Part model, mm, in its own coordinate system. Give positions to 0.01 mm unless a question says otherwise; leave off trailing zeros. Order: outer loops, then holes, each group sorted by start corner. A loop starts at its lowest first (then second) coordinate and runs counter-clockwise, first axis right, second up. Notation, with made-up numbers: M -31.75,37 L 24.25,37 A24 ccw 24.25,50 Z; hole C 75.25,31 d10. An arc over 180 degrees is marked long. Return JSON: item names as keys, results as strings.
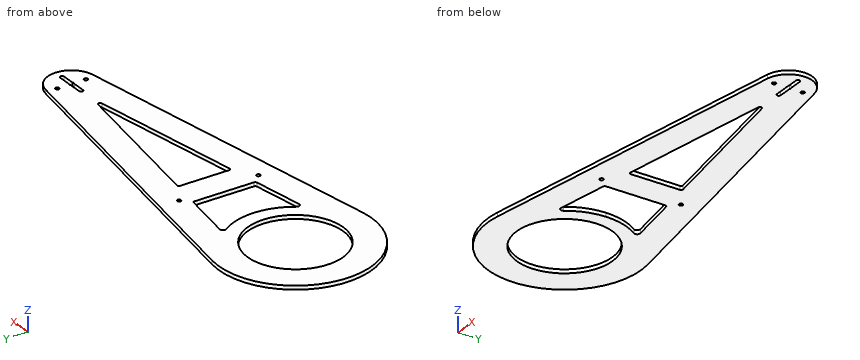
from build123d import *

# Parameters (mm, degrees)
SM_BASE_FLANGE_1_DEPTH = 4
SKETCH_6_R             = 20
SKETCH_6_R_2           = 2.5
CUT_EXTRUDE_1_DEPTH    = 10
SKETCH_7_R             = 2
CUT_EXTRUDE_2_DEPTH    = 10
CUT_EXTRUDE_3_DEPTH    = 10
SKETCH_9_R             = 2
CUT_EXTRUDE_4_DEPTH    = 80
FILLET_2_R             = 2
SKETCH_10_R            = 50
CUT_EXTRUDE_5_DEPTH    = 10


# Sheet-metal steps are written as plain solids
with BuildPart() as part:
    # Sketch 1 → 基体-法兰1 (new body)
    with BuildSketch(Plane.XY):
        with BuildLine():
            Line((12.571428571, 79.00607055), (353.928571429, 24.689397047))
            ThreePointArc((353.928571429, 24.689397047), (375, 0), (353.928571429, -24.689397047))
            Line((353.928571429, -24.689397047), (12.571428571, -79.00607055))
            ThreePointArc((12.571428571, -79.00607055), (-80, 0), (12.571428571, 79.00607055))
        make_face()
    extrude(amount=-SM_BASE_FLANGE_1_DEPTH)

    # 草图6 → 切除-拉伸1 (cut)
    with BuildSketch(Plane.XY):
        Circle(SKETCH_6_R)
        with Locations((350, 0)):
            Circle(SKETCH_6_R_2)
    extrude(amount=-CUT_EXTRUDE_1_DEPTH, mode=Mode.SUBTRACT)

    # 草图7 → 切除-拉伸2 (cut)
    with BuildSketch(Plane.XY):
        with Locations((365, 0)):
            Circle(SKETCH_7_R)
        with Locations((350, -15)):
            Circle(SKETCH_7_R)
        with Locations((335, 0)):
            Circle(SKETCH_7_R)
        with Locations((350, 15)):
            Circle(SKETCH_7_R)
        with BuildLine():
            Line((111.294862901, 32.919806827), (111.294862901, -32.919806827))
            Line((111.294862901, -32.919806827), (56.389238276, -41.656377743))
            ThreePointArc((56.389238276, -41.656377743), (53.378656764, -40.291367953), (53.450847511, -36.986577299))
            ThreePointArc((53.450847511, -36.986577299), (62.032293151, -19.416348946), (64.999939097, -0.088979461))
            ThreePointArc((64.999939097, -0.088979461), (62.058814357, 19.33141383), (53.450847511, 36.986577299))
            ThreePointArc((53.450847511, 36.986577299), (53.378656764, 40.291367953), (56.389238276, 41.656377743))
            Line((56.389238276, 41.656377743), (111.294862901, 32.919806827))
        make_face()
        Polygon((141.940088648, 28.043545246), (141.940088648, -28.043545246), (318.181818182, 0), align=None)
    extrude(amount=-CUT_EXTRUDE_2_DEPTH, mode=Mode.SUBTRACT)

    # 草图8 → 切除-拉伸3 (cut)
    with BuildSketch(Plane.XY):
        with BuildLine():
            Line((347.5, 0), (337, 0))
            ThreePointArc((337, 0), (336.414213562, -1.414213562), (335, -2))
            Line((335, -2), (348.5, -2))
            ThreePointArc((348.5, -2), (347.763932023, -1.118033989), (347.5, 0))
        make_face()
        with BuildLine():
            ThreePointArc((335, 2), (336.414213562, 1.414213562), (337, 0))
            Line((337, 0), (347.5, 0))
            ThreePointArc((347.5, 0), (347.763932023, 1.118033989), (348.5, 2))
            Line((348.5, 2), (335, 2))
        make_face()
        with BuildLine():
            ThreePointArc((351.5, 2), (352.236067977, 1.118033989), (352.5, 0))
            Line((352.5, 0), (363, 0))
            ThreePointArc((363, 0), (363.585786438, 1.414213562), (365, 2))
            Line((365, 2), (351.5, 2))
        make_face()
        with BuildLine():
            Line((363, 0), (352.5, 0))
            ThreePointArc((352.5, 0), (352.236067977, -1.118033989), (351.5, -2))
            Line((351.5, -2), (365, -2))
            ThreePointArc((365, -2), (363.585786438, -1.414213562), (363, 0))
        make_face()
    extrude(amount=-CUT_EXTRUDE_3_DEPTH, mode=Mode.SUBTRACT)

    # 草图9 → 切除-拉伸4 (cut)
    with BuildSketch(Plane.XY):
        with Locations((120, 41.660451514)):
            Circle(SKETCH_9_R)
        with Locations((120, -41.660451514)):
            Circle(SKETCH_9_R)
    extrude(amount=-CUT_EXTRUDE_4_DEPTH, mode=Mode.SUBTRACT)

    # 圆角2
    fillet_2_edges = [part.edges().sort_by_distance(p)[0] for p in [
        (141.940088648, 28.043545246, -2),
        (318.181818182, 0, -2),
        (141.940088648, -28.043545246, -2),
        (111.294862901, 32.919806827, -2),
        (111.294862901, -32.919806827, -2),
    ]]
    fillet(fillet_2_edges, radius=FILLET_2_R)

    # 草图10 → 切除-拉伸5 (cut)
    with BuildSketch(Plane.XY):
        Circle(SKETCH_10_R)
    extrude(amount=-CUT_EXTRUDE_5_DEPTH, mode=Mode.SUBTRACT)


solid = part.part
Q1. Band-saw the part on C-C (x = 207). Give the cut face in (y, z), then the cut area to 3 significant figures.
Established:
{"outline": "M -48.07,-4 L -17.69,-4 L -17.69,0 L -48.07,0 Z; M 17.69,-4 L 48.07,-4 L 48.07,0 L 17.69,0 Z", "area": "243 mm²"}
Q2. Band-saw the part on D-D (y = 69). Give the cut face in (x, z).
Established:
{"outline": "M -40.48,-4 L 75.46,-4 L 75.46,0 L -40.48,0 Z"}
Q3. Band-saw the part on B-B (z = -2.35). Give the number of separate pieces and of enclosed holes in the cut face, then the cut area to 3 significant figures.
Established:
{"separate pieces": "1", "enclosed holes": "8", "area": "31,500 mm²"}
Q4. Band-saw the part on A-A (x = 0). Give the cut face in (y, z), then the cut area to 3 significant figures.
Established:
{"outline": "M -80,-4 L -50,-4 L -50,0 L -80,0 Z; M 50,-4 L 80,-4 L 80,0 L 50,0 Z", "area": "240 mm²"}
Q5. Probe line 1 along Y through (x, z) = (120, -0.95); line 2 along Y through (x, z) = (350, -2.9); line 3 along Y through (x, z) = (3.5, -3.4). List the from-to ranges inside material, lowest first.
Established:
{"line 1": "y = -61.91 to -43.66, -39.66 to 39.66, 43.66 to 61.91", "line 2": "y = -25.31 to -17, -13 to -2.5, 2.5 to 13, 17 to 25.31", "line 3": "y = -79.92 to -49.88, 49.88 to 79.92"}
Q6. Pin check, flat tips, straight feed: pin 1 (2 mm diameter, centred on y = 21, z = -2, fed in from -X); pin 2 (1.2 mm diameter, centred on x = 356, z = -1.5, fed in from -Y); pin 3 (3.5 mm diameter, centred on x = 120, y = -41.66, fed in from -Z); pin 4 (2 mm diameter, centred on x = 340.5, z = -1.5, fed in from -Y). Stop position of each tip, or through.
Established:
{"pin 1": "stops at x = -77.46", "pin 2": "stops at y = -24.41", "pin 3": "passes through", "pin 4": "stops at y = -26.99"}
